Work out the finished part from the listing and answer in its coordinate system (mm). Round coordinates to 2 decimals unless told otherwise and drop trailing zeros. Write each loop counter-clockwise with the first axis right and the second up, starting at its lowest first coordinate (ties: lowest second). Pieces come first, ordered by that corner, then holes.
1. Find section B-B (z = 9). Write down the section's boundary in (x, y) (3 decimals).
2. Straight lines are drawn through the part: probe 1 along Z at (x, y) = (-4, -7.25); probe 2 along Z at (x, y) = (-5.5, -9.25); probe 3 along X at (y, z) = (-3, 11.25). For each, find the intervals that lie inside material, in ascending order.
3. Find section A-A (y = -11). Write down the section's boundary in (x, z), and give its area (3 significant figures).
4. Find section C-C (x = -3.5). Write down the section's boundary in (y, z).
```python
from build123d import *

# Parameters (mm, degrees)
F0_W     = 9
F0_H     = 12.4
F1_DEPTH = 4
F2_W     = 9
F2_H     = 12.4
F3_DEPTH = 4
F5_DEPTH = 12.4
F6_R     = 1


with BuildPart() as f1:
    # F0 (on Top) → F1 (new body)
    with BuildSketch(Plane.XY):
        with Locations((-4.5, -6.2)):
            Rectangle(F0_W, F0_H)
    extrude(amount=F1_DEPTH)

    # F2 (on face) → F3 (join)
    with BuildSketch(Plane.XY.offset(4)):
        with Locations((-4.5, -6.2)):
            Rectangle(F2_W, F2_H)
    extrude(amount=F3_DEPTH)

    # F4 (on face) → F5 (join, through all)
    with BuildSketch(Plane.XZ.offset(12.4)):
        Polygon((-4.5, 12), (-9, 8), (0, 8), align=None)
    extrude(amount=-F5_DEPTH)

    # F6
    f6_edges = [f1.edges().sort_by_distance(p)[0] for p in [
        (-4.5, -6.2, 12),
    ]]
    fillet(f6_edges, radius=F6_R)


solid = f1.part
```
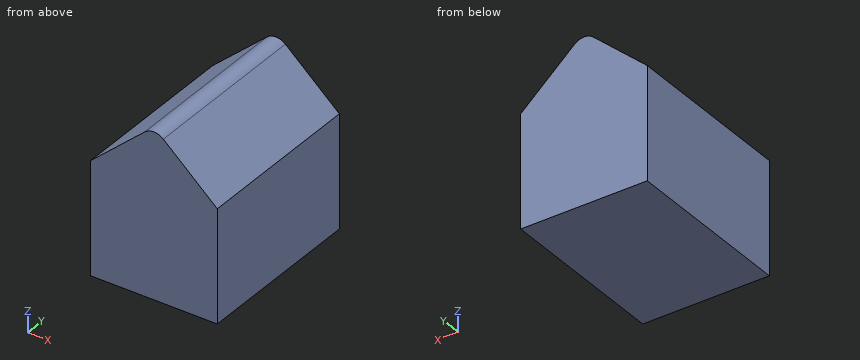
Worked answers:
1. outline: (-7.875, -12.4) - (-1.125, -12.4) - (-1.125, 0) - (-7.875, 0) - close
2. probe 1: z = 0 to 11.53
2. probe 2: z = 0 to 11.11
2. probe 3: x = -5.34 to -3.66
3. outline: (-9, 0) - (0, 0) - (0, 8) - (-3.84, 11.41) arc R1 ccw to (-5.16, 11.41) - (-9, 8) - close
3. area: 89.8 mm2
4. outline: (-12.4, 0) - (0, 0) - (0, 11.11) - (-12.4, 11.11) - close
